```python
from build123d import *

# Parameters (mm, degrees)
BOSS_EXTRU_1_DEPTH = 3


with BuildPart() as part:
    # Esquisse1 → Boss.-Extru.1 (new body)
    with BuildSketch(Plane.XY):
        Polygon((71.175872824, -27.390104167), (71.175872824, -7.390104167), (68.175872824, -7.390104167), (68.175872824, 22.609895833), (71.175872824, 22.609895833), (71.175872824, 29.609895833), (41.175872824, 29.609895833), (41.175872824, 32.609895833), (11.175872824, 32.609895833), (11.175872824, 29.609895833), (-18.824127176, 29.609895833), (-18.824127176, 32.609895833), (-48.824127176, 32.609895833), (-48.824127176, 29.609895833), (-78.824127176, 29.609895833), (-78.824127176, 22.609895833), (-75.824127176, 22.609895833), (-75.824127176, -7.390104167), (-78.824127176, -7.390104167), (-78.824127176, -27.390104167), (-75.824127176, -27.390104167), (-75.824127176, -57.390104167), (-78.824127176, -57.390104167), (-78.824127176, -64.390104167), (-48.824127176, -64.390104167), (-48.824127176, -67.390104167), (-18.824127176, -67.390104167), (-18.824127176, -64.390104167), (11.175872824, -64.390104167), (11.175872824, -67.390104167), (41.175872824, -67.390104167), (41.175872824, -64.390104167), (71.175872824, -64.390104167), (71.175872824, -57.390104167), (68.175872824, -57.390104167), (68.175872824, -27.390104167), align=None)
    extrude(amount=BOSS_EXTRU_1_DEPTH)


solid = part.part
```
The listing builds one solid part. Answer for the finished solid, in the listing's coordinates (mm). A direction names the side the tool comes from. Round coordinates to 2 decimals unless told otherwise and drop trailing zeros. Loops run counter-clockwise (first coordinate to the right, second up) from the corner with the lowest first, then second, coordinate; pieces in that order, holes last.
Q1. Find the intervals of material crossed by line 1 (X direction, y = 6, z = 2.45); line 2 (Y direction, x = 61.5, z = 0.35), in increasing order.
Q2. Section A-A, the plane y = -3 is taken. Determine the outline of the cut face in (x, z), then the cut area to 3 significant figures.
Q3. Which of the six approach directions +Z, -Z, +X, -X, +Y, -Y give full straight-line access (tool end or side, diameter ignored) to faces 1 (the face through (-18.824, -66, 1)), 2 (the face through (70, -7.39, 1)), 3 (the face through (56, 29.61, 1))?
Q4. Section B-B, the plane x = 6 is taken. Determine the outline of the cut face in (y, z), then the cut area to 3 significant figures.
Q5. For a pull along X with two mould halves and no side action, classify faces 4 (the face through (-78.824, 26, 1)), 5 (the face through (-18.824, 31, 1)), 6 (the face through (41.176, -66, 1)) as released by +X, released by -X, zero draft, split by the parting line, or undercut.
Q6. Given pin 1 Ø1.5 at (x, z) = (-62, 1) entering from +Y; pin 2 Ø0.9 at (x, z) = (52, 1) entering from -Y; pin 3 Ø1.5 at (y, z) = (11.5, 2) entering from -X, each flat-ended and moving along its own axis, determine where each tip first touches the part or whether it passes through.
Completed:
1. line 1: x = -75.82 to 68.18
1. line 2: y = -64.39 to 29.61
2. outline: (-75.82, 0) - (68.18, 0) - (68.18, 3) - (-75.82, 3) - close
2. area: 432 mm2
3. face 1: +Z, -Z, -Y
3. face 2: +Z, -Z, +X
3. face 3: +Z, -Z, +X, +Y
4. outline: (-64.39, 0) - (29.61, 0) - (29.61, 3) - (-64.39, 3) - close
4. area: 282 mm2
5. face 4: released by -X
5. face 5: undercut
5. face 6: released by +X
6. pin 1: stops at y = 29.61
6. pin 2: stops at y = -64.39
6. pin 3: stops at x = -75.82
